Design review of the part shown in the three views and the two pictorial views. Dimensions are in mm from the part's minimum x, y and z. Give positions to 0.01 mm unless a question says otherwise; leave off trailing zeros. Loops run counter-clockwise (first coordinate to the right, second up) from the corner with the lowest first, then second, coordinate; pieces in that order, holes last.
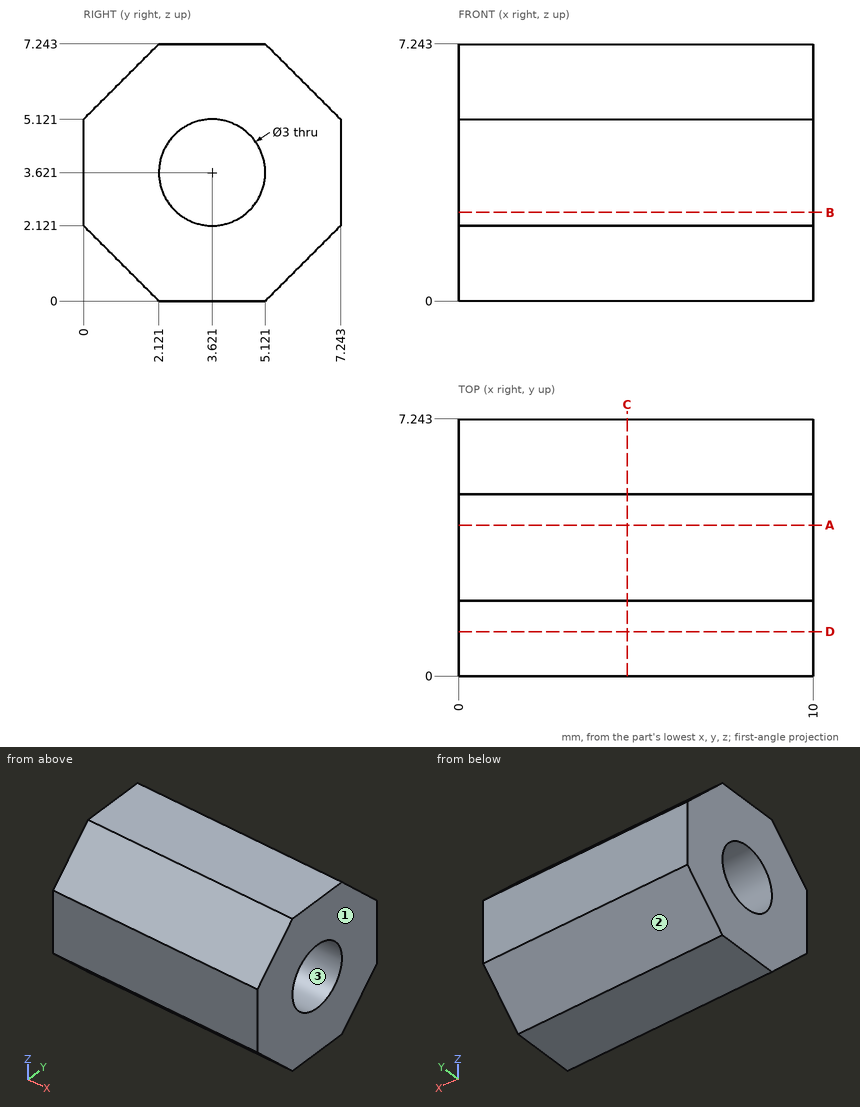
Q1. Take a section at A-A (y = 4.25). Give the boundary of the cut face in (x, z).
Results:
outline: (0, 0) - (10, 0) - (10, 2.26) - (0, 2.26) - close; (0, 4.98) - (10, 4.98) - (10, 7.24) - (0, 7.24) - close
Q2. Wall thickness on line 1 (Z direction, x = 0.75, y = 4.75) (1 decimal); line 2 (Z direction, x = 5, y = 4); line 3 (Y direction, x = 9.5, z = 3) (1 decimal): over which ranges is each line inside the solid? List them lowest first.
Results:
line 1: z = 0 to 2.6, 4.6 to 7.2
line 2: z = 0 to 2.17, 5.07 to 7.24
line 3: y = 0 to 2.3, 5 to 7.2
Q3. Take a section at B-B (z = 2.5). Give the boundary of the cut face in (x, y) (1 decimal), plus the area to 3 significant figures.
Results:
outline: (0, 0) - (10, 0) - (10, 2.6) - (0, 2.6) - close; (0, 4.6) - (10, 4.6) - (10, 7.2) - (0, 7.2) - close
area: 52.5 mm2
Q4. Draft analysis for pull direction Z (two halves, no side actions). For the marked faces 1, 2 and 3, state which applies: pulls with the +Z half, pulls with the -Z half, needs draft (parallel to the pull), parting line crosses it, or undercut.
Results:
face 1: needs draft
face 2: pulls with the -Z half
face 3: undercut
Q5. Take a section at D-D (y = 1.25). Give the boundary of the cut face in (x, z).
Results:
outline: (0, 0.87) - (10, 0.87) - (10, 6.37) - (0, 6.37) - close
Q6. Take a section at C-C (x = 4.75). Give the boundary of the cut face in (y, z), plus the area to 3 significant figures.
Results:
outline: (0, 2.12) - (2.12, 0) - (5.12, 0) - (7.24, 2.12) - (7.24, 5.12) - (5.12, 7.24) - (2.12, 7.24) - (0, 5.12) - close; hole circle Ø3 at (3.62, 3.62)
area: 36.4 mm2
Q7. Insertion check: pin 1 (3 mm diameter, centred on x = 4, y = 5.5, fed in from -Z); pin 2 (1.5 mm diameter, centred on x = 7, y = 6, fed in from -Z). Each pin has a flat end and moves straight along its axis. Give the tip position at first contact, or say it passes through.
Results:
pin 1: stops at z = 0
pin 2: stops at z = 0.13
